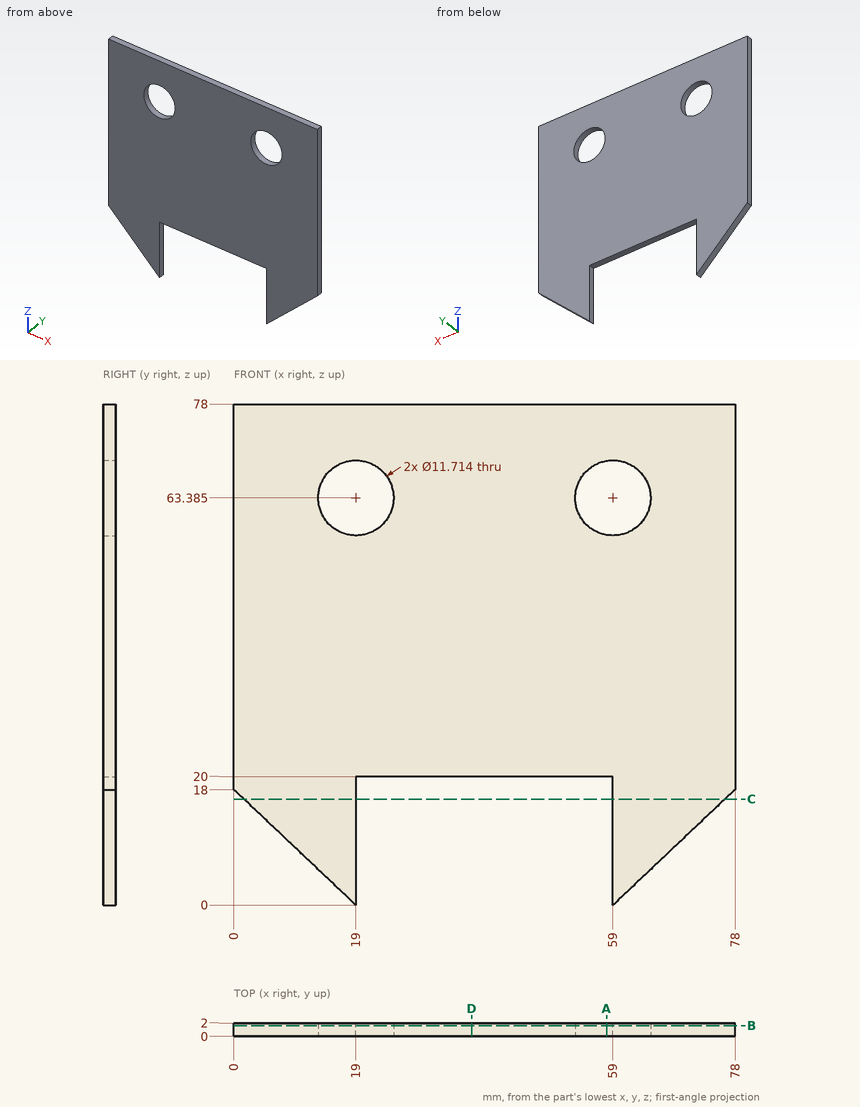
For this review, use the dimensioned drawing (mm, ordinates from the lowest corner) and the shaded views. Give positions to 0.01 mm unless a question says otherwise; leave off trailing zeros. Order: outer loops, then holes, each group sorted by start corner. A loop starts at its lowest first (then second) coordinate and runs counter-clockwise, first axis right, second up. Notation, with made-up numbers: M 12.5,23 L 60.5,23 A23 ccw 60.5,39 Z; hole C -14.75,44.5 d10. An arc over 180 degrees is marked long. Use one line per item in the form item = value. Start each with the question number.
Item 1: We need section C-C on z = 16.5. Give the boundary of the cut face in (x, y).
Item 2: We need section A-A on x = 58. Give the boundary of the cut face in (y, z) (1 decimal).
Item 3: To check wall thickness, follow line 1 along X through (y, z) = (1.15, 63) (1 decimal); line 2 along X through (y, z) = (0.4, 61); line 3 along Z through (x, y) = (43, 1.75). State the ranges of each line that lie inside material, in increasing order. Write a range as from..to.
Item 4: We need section B-B on y = 1.6. Give the boundary of the cut face in (x, z) (1 decimal).
Item 5: We need section D-D on x = 37. Give the boundary of the cut face in (y, z), plus the area to 3 significant figures.
Completed:
q1.outline = M 1.58,0 L 19,0 L 19,2 L 1.58,2 Z; M 59,0 L 76.42,0 L 76.42,2 L 59,2 Z
q2.outline = M 0,20 L 2,20 L 2,57.6 L 0,57.6 Z; M 0,69.2 L 2,69.2 L 2,78 L 0,78 Z
q3.line_1 = 0..13.2, 24.8..53.2, 64.8..78
q3.line_2 = 0..13.65, 24.35..53.65, 64.35..78
q3.line_3 = 20..78
q4.outline = M 0,18 L 19,0 L 19,20 L 59,20 L 59,0 L 78,18 L 78,78 L 0,78 Z; hole C 19,63.4 d11.7; hole C 59,63.4 d11.7
q5.outline = M 0,20 L 2,20 L 2,78 L 0,78 Z
q5.area = 116 mm²
